Here's how the part is built. I have some questions about the finished solid (model axes, mm). A direction names the side the tool comes from. Coordinates: 2 decimals unless noted, no trailing zeros. Loops run counter-clockwise (first coordinate to the right, second up) from the corner with the lowest first, then second, coordinate; pieces in that order, holes last.
Autodesk Inventor part; units mm, degrees
ref_plane "YZ Plane" through (0, 0, 0) normal (1, 0, 0) x (0, 1, 0)
ref_plane "XZ Plane" through (0, 0, 0) normal (0, 1, 0) x (-1, 0, 0)
ref_plane "XY Plane" through (0, 0, 0) normal (0, 0, 1) x (1, 0, 0)
sketch "Boceto1" plane through (0, 0, 0) normal (0, 0, 1) x (1, 0, 0)
  line L0 (-20, 20) -> (20, 20)
  line L1 (20, 20) -> (20, -20)
  line L2 (20, -20) -> (-20, -20)
  line L3 (-20, -20) -> (-20, 20)
  line L4 (-20, 20) -> (20, -20) construction
  line L5 (-16, 16) -> (16, 16)
  line L6 (16, 16) -> (16, -16)
  line L7 (16, -16) -> (-16, -16)
  line L8 (-16, -16) -> (-16, 16)
  line L9 (-16, 0) -> (-20, 0) construction
  line L10 (0, 16) -> (0, 20) construction
  line L11 (16, 0) -> (20, 0) construction
  line L12 (0, -16) -> (0, -20) construction
  point P0 (0, 0)
  point P1 (0, 0)
  dimension "d0" = 40
  dimension "d1" = 4
extrude "Extrusión1" add sketch "Boceto1" along normal blind 164
sketch "Boceto2" plane through (20, -20, 0) normal (1, 0, 0) x (0, 0, -1)
  line L0 (0, 20) -> (-164, 20)
  line L1 (-164, 36) -> (-164, 4)
  line L2 (0, 0) -> (0, 40)
  circle A0 centre (-82, 20) radius 16
  point P0 (0, 20)
  dimension "d4" = 32
extrude "Extrusión2" cut sketch "Boceto2" against normal up to surface (4 mm away)
properties part number "C_358_40_2"
1. I want a section at B-B (x = -6.5). Please give me the cut outline in (y, z), then the cut area to 3 significant figures.
2. I want a section at D-D (z = 91.5). Please give me the cut outline in (x, y).
3. For pin 1 (19 mm diameter, centred on y = 0, z = 82, fed in from +X), with a flat end and sliding along its axis, tell me the tip position at first contact or that it passes through.
4. I want a section at A-A (y = 0). Please give me the cut outline in (x, z), then the cut area to 3 significant figures.
5. We'd pull the mould along X, two halves only. Please class faces 4 (the flat face through (-20, 0, 81)), 5 (the flat face through (0, 20, 81)), 6 (the flat face through (16, 0, 132)): +X half, -X half, draft (parallel to the pull), parting line (faces both ways), or undercut.
6. I want a section at C-C (z = 33.5). Please give me the cut outline in (x, y), then the cut area to 3 significant figures.
7. On a 3-axis mill with a long thin cutter (end or side, diameter ignored), from which of +Z, -Z, +X, -X, +Y, -Y can I reach the whole of each face in a straight line? I mean faces 1 (the flat face through (-18, 0, 0)), 2 (the cylindrical face through (18.028, -9.736, 94.697)), 3 (the flat face through (16, 0, 31)). Say none if no direction works.
8. I need wall thicknesses on line 1 along Y through (x, z) = (18.55, 82); line 2 along Z through (x, y) = (18, 0). Which ranges of each line are inside material? Lowest first, please.
Response values:
1. outline: (-20, 0) - (-16, 0) - (-16, 164) - (-20, 164) - close; (16, 0) - (20, 0) - (20, 164) - (16, 164) - close
1. area: 1,310 mm2
2. outline: (-20, -20) - (20, -20) - (20, -12.87) - (16, -12.87) - (16, -16) - (-16, -16) - (-16, 16) - (16, 16) - (16, 12.87) - (20, 12.87) - (20, 20) - (-20, 20) - close
3. pin 1: stops at x = -16
4. outline: (-20, 0) - (-16, 0) - (-16, 164) - (-20, 164) - close; (16, 0) - (20, 0) - (20, 66) - (16, 66) - close; (16, 98) - (20, 98) - (20, 164) - (16, 164) - close
4. area: 1,180 mm2
5. face 4: -X half
5. face 5: draft
5. face 6: undercut
6. outline: (-20, -20) - (20, -20) - (20, 20) - (-20, 20) - close; hole (-16, -16) - (16, -16) - (16, 16) - (-16, 16) - close
6. area: 576 mm2
7. face 1: -Z, +X, -X, +Y, -Y
7. face 2: +X
7. face 3: +Z, -Z
8. line 1: y = -20 to -16, 16 to 20
8. line 2: z = 0 to 66, 98 to 164
